Geometry check sheet. Reference: the model listing, model coordinates, mm. A direction names the side the tool comes from. Round coordinates to 2 decimals unless told otherwise and drop trailing zeros. Write each loop counter-clockwise with the first axis right and the second up, starting at its lowest first coordinate (ties: lowest second). Pieces come first, ordered by that corner, then holes. Notation, with made-up numbers: M -6.75,17 L 5.25,17 A15 cw 5.25,27 Z; hole C 26,0 d9. An arc over 180 degrees is marked long. Put each result on its own line as item: value. Start each with the question number.
(1) Section check D-D on y = 8. Record the cut outline in (x, z).
(2) Gauge pin test, flat ends, axial feed: pin 1 (5 mm diameter, centred on y = 9.5, z = 15, fed in from +X); pin 2 (4 mm diameter, centred on x = 17.5, y = -22.5, fed in from -Z); pin 3 (12 mm diameter, centred on x = 27, y = 10.5, fed in from -Z). Record the tip position at first contact, or that the pin passes through.
(3) Material ranges on probe 1 along Z at (x, y) = (0, 34); probe 2 along X at (y, z) = (-28, 15.5); probe 3 along X at (y, z) = (-2, 12), recorded low to high.
(4) Section check C-C on z = -22.5. Record the cut outline in (x, y).
(5) Section check B-B on x = 5. Record the cut outline in (y, z), then the cut area to 3 significant figures.
(6) Mould release check, pull along X, two halves, no side actions. Record for faces 3 (the flat face through (0, 0, -46.044)), 4 (the cylindrical face through (11.23, 3.93, 50.57)), 5 (the cylindrical face through (-28.174, 2.898, 14.466)): pulls with the +X half, pulls with the -X half, needs draft (parallel to the pull), parting line crosses it, or undercut.
(7) Tool access check on faces 1 (the flat face through (0.721, -8.965, -20.912)), 2 (the cylindrical face through (22.12, 2.9, 12.26)). Record the directions out of +Z, -Z, +X, -X, +Y, -Y that give a thin tool (end or side, any length) a straight path to the whole face; none if there is none.
(8) Section check A-A on y = -20. Record the cut outline in (x, z).
from build123d import *

# Parameters (mm, degrees)
F0_W          = 51.8020391464
F0_H          = 74.018985033
F3_D          = 6.7564
F5_DEPTH      = 51.8030391464
F5_DEPTH_BACK = 51.8030391464


with BuildPart() as f1:
    # F0 (on Top) → F1 (revolve)
    with BuildSketch(Plane.XY):
        with Locations((-25.9010195732, 3.415748477)):
            Rectangle(F0_W, F0_H)
    revolve(axis=Axis((0, 3.415748477, 0), (0, -1, 0)))

    # F3 (through all)
    with Locations(Plane(origin=(0, 40.4252409935, 0), x_dir=(-1, 0, 0), z_dir=(0, 1, 0))):
        with Locations((-24.7987365379, 14.3175572157), (0, -28.6351144314), (24.7987365379, 14.3175572157)):
            Hole(F3_D / 2)

    # F4 (on Right) → F5 (cut, two sides)
    with BuildSketch(Plane.YZ) as f5_sk:
        Polygon((-23.4744153275, -46.0438393056), (23.4744153275, -46.0438393056), (0, -5.3849592805), align=None)
    extrude(amount=F5_DEPTH, mode=Mode.SUBTRACT)
    extrude(f5_sk.sketch, amount=-F5_DEPTH_BACK, mode=Mode.SUBTRACT)


solid = f1.part
Answers follow:
1. outline: M -48.1,-19.24 L 48.1,-19.24 A51.8 ccw long Z; M -23.74,-46.04 A51.8 ccw 23.74,-46.04 Z; hole C -24.8,14.32 d6.76; hole C 24.8,14.32 d6.76
2. pin 1: stops at x = 50.27
2. pin 2: stops at z = -49.43
2. pin 3: stops at z = -47.35
3. probe 1: z = -51.8 to -32.01, -25.26 to 51.8
3. probe 2: x = -49.43 to -27.96, -21.63 to 21.63, 27.96 to 49.43
3. probe 3: x = -50.39 to -27.26, -22.34 to 22.34, 27.26 to 50.39
4. outline: M -46.66,-33.59 L 46.66,-33.59 L 46.66,-9.88 L -46.66,-9.88 Z; M -46.66,9.88 L 46.66,9.88 L 46.66,40.43 L -46.66,40.43 Z
5. outline: M -33.59,-51.56 L 40.43,-51.56 L 40.43,51.56 L -33.59,51.56 Z; hole M -23.47,-46.04 L 23.47,-46.04 L 0,-5.38 Z
5. area: 6,680 mm^2
6. face 3: needs draft
6. face 4: parting line crosses it
6. face 5: undercut
7. face 1: +X, -X
7. face 2: +Y, -Y
8. outline: M -32.88,-40.03 L 32.88,-40.03 A51.8 ccw long Z; M -23.74,-46.04 A51.8 ccw 23.74,-46.04 Z; hole C -24.8,14.32 d6.76; hole C 0,-28.64 d6.76; hole C 24.8,14.32 d6.76
